CAD build for the part. Positions are in the model's coordinates, mm. A direction names the side the tool comes from. Give positions to 0.01 mm unless a question says otherwise; leave off trailing zeros. Write each loop counter-clockwise with the first axis right and the second up, starting at its lowest first coordinate (ties: lowest second). Pieces come first, ordered by that corner, then holes. Notation, with made-up numbers: M 27,68 L 45,68 A21 ccw 45,95 Z; hole C -15.75,-9.75 d9. An arc over 180 degrees is marked long. One line per question, with ' | ' between items. Start each with the question number.
1. Cut at A-A, the plane z = 20. Write the cut outline in (x, y), then the cut area to 3 significant figures.
2. Cut at B-B, the plane x = 19.25. Write the cut outline in (y, z).
3. Which spindle directions (+Z, -Z, +X, -X, +Y, -Y) get a long thin tool onto all of the face, cutting with end or side? Do faces 1 (the face through (16.022, -47.647, 29.052)), 2 (the face through (38.743, 62, 28)). Say none if no direction does.
4. Wall check: L1, parallel to Y at x = 23.5, z = 13; L2, parallel to Y at x = 33.5, z = 55.5; L3, parallel to X at y = 43.5, z = 47. Give the ranges that are in metal, low to high.
5. Pull direction Y, two halves, no side cores. Call faces 3 (the face through (35.172, 56.979, 28.25)), 4 (the face through (38.743, -50, 28)), 5 (the face through (15.14, -51.65, 29.05)): released by +Y, released by -Y, zero draft, split by the parting line, or undercut.
6. Cut at C-C, the plane y = -2.5. Write the cut outline in (x, z).
7. Flat gauge pins, fed straight in: pin 1 (12 mm diameter, centred on y = 39, z = 34, fed in from +X); pin 2 (3 mm diameter, centred on x = 20.5, z = 27.5, fed in from -Y); pin 3 (0.5 mm diameter, centred on y = -45.5, z = 41.5, fed in from -X). Where does each tip first touch, or does it go through?
```python
from build123d import *

# Parameters (mm, degrees)
SKETCH1_R           = 2.62509
SKETCH1_R_2         = 2.6289
BOSS_EXTRUDE1_DEPTH = 57.3024
FILLET1_R           = 2.54
FILLET2_R           = 1
FILLET3_R           = 10.16


with BuildPart() as part:
    # Sketch1 → Boss-Extrude1 (new body)
    with BuildSketch(Plane.XY):
        with BuildLine():
            Line((26.744137004, -45.371617498), (26.744137004, -48.371357498))
            Line((26.744137004, -48.371357498), (15.258617004, -48.371357498))
            Line((15.258617004, -48.371357498), (15.258617004, 60.986122502))
            Line((15.258617004, 60.986122502), (26.744137004, 60.986122502))
            Line((26.744137004, 60.986122502), (26.744137004, 57.986382502))
            ThreePointArc((26.744137004, 57.986382502), (32.743617004, 51.986902502), (38.743097004, 57.986382502))
            Line((38.743097004, 57.986382502), (38.743097004, 67.160862502))
            Line((38.743097004, 67.160862502), (32.743617004, 67.160862502))
            Line((32.743617004, 67.160862502), (12.083617004, 67.160862502))
            Line((12.083617004, 67.160862502), (12.083617004, -54.546097498))
            Line((12.083617004, -54.546097498), (32.743617004, -54.546097498))
            Line((32.743617004, -54.546097498), (38.743097004, -54.546097498))
            Line((38.743097004, -54.546097498), (38.743097004, -45.371617498))
            ThreePointArc((38.743097004, -45.371617498), (32.743617004, -39.372137498), (26.744137004, -45.371617498))
        make_face()
        with Locations((32.743617004, -45.371617498)):
            Circle(SKETCH1_R, mode=Mode.SUBTRACT)
        with Locations((32.743617004, 57.986382502)):
            Circle(SKETCH1_R_2, mode=Mode.SUBTRACT)
    extrude(amount=BOSS_EXTRUDE1_DEPTH)

    # Fillet1
    fillet1_edges = [part.edges().sort_by_distance(p)[0] for p in [
        (26.744137004, 60.986122502, 28.6512),
        (15.258617004, 60.986122502, 28.6512),
        (15.258617004, -48.371357498, 28.6512),
        (26.744137004, -48.371357498, 28.6512),
    ]]
    fillet(fillet1_edges, radius=FILLET1_R)

    # Fillet2
    fillet2_edges = [part.edges().sort_by_distance(p)[0] for p in [
        (38.743097004, -54.546097498, 28.6512),
        (38.743097004, 67.160862502, 28.6512),
    ]]
    fillet(fillet2_edges, radius=FILLET2_R)

    # Fillet3
    fillet3_edges = [part.edges().sort_by_distance(p)[0] for p in [
        (12.083617004, -54.546097498, 28.6512),
    ]]
    fillet(fillet3_edges, radius=FILLET3_R)


solid = part.part
```
Here are the results:
1) outline: M 12.08,-44.39 A10.16 ccw 22.24,-54.55 L 37.74,-54.55 A1 ccw 38.74,-53.55 L 38.74,-45.37 A6 ccw 26.74,-45.37 L 26.74,-45.83 A2.54 cw 24.2,-48.37 L 17.8,-48.37 A2.54 cw 15.26,-45.83 L 15.26,58.45 A2.54 cw 17.8,60.99 L 24.2,60.99 A2.54 cw 26.74,58.45 L 26.74,57.99 A6 ccw 38.74,57.99 L 38.74,66.16 A1 ccw 37.74,67.16 L 12.08,67.16 Z; hole C 32.74,57.99 d5.26; hole C 32.74,-45.37 d5.25 | area: 801 mm^2
2) outline: M -54.1,0 L -48.37,0 L -48.37,57.3 L -54.1,57.3 Z; M 60.99,0 L 67.16,0 L 67.16,57.3 L 60.99,57.3 Z
3) face 1: +Z, -Z | face 2: +Z, -Z, +X, +Y, -Y
4) L1: -54.55 to -48.37, 60.99 to 67.16 | L2: -54.55 to -47.89, -42.86 to -39.42, 52.03 to 55.47, 60.5 to 67.16 | L3: 12.08 to 15.26
5) face 3: undercut | face 4: zero draft | face 5: released by -Y
6) outline: M 12.08,0 L 15.26,0 L 15.26,57.3 L 12.08,57.3 Z
7) pin 1: x = 15.26 | pin 2: y = -54.54 | pin 3: x = 12.12
